from build123d import *

# Parameters (mm, degrees)
F1_DEPTH = 10
F3_DEPTH = 10
F4_SIZE2 = 8.660244
F4_SIZE  = 4.99999
F5_R     = 5


# Not quite as in the source:
# - a fillet or chamfer is up to 0.001 mm smaller than in the source, because OpenCascade refuses the exact size


with BuildPart() as f1:
    # F0 (on Front) → F1 (new body)
    with BuildSketch(Plane.XZ):
        with BuildLine():
            Line((0.8717797887, -2.5), (7.5, -2.5))
            Line((7.5, -2.5), (7.5, 2.5))
            Line((7.5, 2.5), (-7.5, 2.5))
            Line((-7.5, 2.5), (-7.5, -2.5))
            Line((-7.5, -2.5), (-0.8717797887, -2.5))
            ThreePointArc((-0.8717797887, -2.5), (0, 1.3), (0.8717797887, -2.5))
        make_face()
    extrude(amount=F1_DEPTH)

    # F2 (on face) → F3 (join)
    with BuildSketch(Plane(origin=(0, 0, 0), x_dir=(-1, 0, 0), z_dir=(0, 1, 0))):
        with BuildLine():
            ThreePointArc((0.8717797887, -2.5), (0, 1.3), (-0.8717797887, -2.5))
            Line((-0.8717797887, -2.5), (0.8717797887, -2.5))
        make_face()
        with BuildLine():
            Line((7.5, 2.5), (-7.5, 2.5))
            Line((-7.5, 2.5), (-7.5, -2.5))
            Line((-7.5, -2.5), (-0.8717797887, -2.5))
            ThreePointArc((-0.8717797887, -2.5), (0, 1.3), (0.8717797887, -2.5))
            Line((0.8717797887, -2.5), (7.5, -2.5))
            Line((7.5, -2.5), (7.5, 2.5))
        make_face()
    extrude(amount=F3_DEPTH)

    # F4 (size 5 and 8.6602540378 in the source; OpenCascade refuses exactly that, so slightly less here)
    f4_edges = [f1.edges().sort_by_distance(p)[0] for p in [
        (0, 10, -2.5),
    ]]
    f4_side = f1.faces().sort_by_distance((0, 10, 0))[0]
    chamfer(f4_edges, length=F4_SIZE, length2=F4_SIZE2, reference=f4_side)

    # F5
    f5_edges = [f1.edges().sort_by_distance(p)[0] for p in [
        (0, 1.339756, -2.5),
        (7.5, 5.669878, -5e-06),
        (-7.5, 5.669878, -5e-06),
    ]]
    fillet(f5_edges, radius=F5_R)


solid = f1.part
Here's how the part is built. I have some questions about the finished solid (model axes, mm). A direction names the side the tool comes from. Round coordinates to 2 decimals unless told otherwise and drop trailing zeros. Order: outer loops, then holes, each group sorted by start corner. A loop starts at its lowest first (then second) coordinate and runs counter-clockwise, first axis right, second up. Notation, with made-up numbers: M 0.25,17 L 18.25,17 A6 cw 18.25,24 Z; hole C 2.25,-25.75 d11. An arc over 180 degrees is marked long. Return JSON: item names as keys, results as strings. Group by question number.
1. If we mould it in two halves opening along Z, with no side actions, what happens to faces 3 (the face through (-0.08, -4.93, 1.3)), 4 (the face through (5.996, 2.889, 0.041)), 5 (the face through (0, 0, 2.5))? For each: pulls with the +Z half, pulls with the -Z half, needs draft (parallel to the pull), parting line crosses it, or undercut.
2. On a 3-axis mill with a long thin cutter (end or side, diameter ignored), from which of +Z, -Z, +X, -X, +Y, -Y can I reach the whole of each face in a straight line? I mean faces 1 (the face through (0, 0, -1)), 2 (the face through (0.035, 6.198, 0.305)). Say none if no direction works.
3. I'm going to push flat-ended pins straight in: pin 1 Ø3 at (x, z) = (0, -0.7) entering from -Y; pin 2 Ø1.5 at (y, z) = (5.5, 0) entering from -X; pin 3 Ø1 at (y, z) = (0, 0) entering from +X. Where does each tip first touch, or does it pass through?
4. Please list where these lines run through material, in increasing order: probe 1 along X at (y, z) = (-7.25, -0.65); probe 2 along X at (y, z) = (-2, -0.8); probe 3 along Y at (x, z) = (-4.75, -1.05).
5. If we section it at B-B on x = 2.75: List the corners of the cut face in (y, z) for me, then the cut area to 3 significant figures.
Reply:
{
 "1": {"face 3": "undercut", "face 4": "pulls with the -Z half", "face 5": "pulls with the +Z half"},
 "2": {"face 1": "-Y", "face 2": "-Z, +X, -X, +Y"},
 "3": {"pin 1": "y = 0", "pin 2": "x = -5.27", "pin 3": "x = 7.21"},
 "4": {"probe 1": "-7.5 to -2, 2 to 7.5", "probe 2": "-7.14 to -2, 2 to 7.14", "probe 3": "-10 to 2.78"},
 "5": {"outline": "M -10,-2.5 L 0,-2.5 A5 ccw 2.28,-1.95 L 9.99,2.5 L -10,2.5 Z", "area": "78.1 mm^2"}
}
